The listing builds one solid part. Answer for the finished solid, in the listing's coordinates (mm). Face numbers are marked on the shaded views. A direction names the side the tool comes from. Round coordinates to 2 decimals unless told otherwise and drop trailing zeros. Order: outer loops, then holes, each group sorted by start corner. A loop starts at its lowest first (then second) coordinate and runs counter-clockwise, first axis right, second up. Notation, with made-up numbers: (-20.75, -12) -> (35.25, -12) arc R21 cw to (35.25, 17) -> close; hole circle Ø4 at (3, 56). An arc over 180 degrees is marked (long way). Answer in a Markdown table with one row per item. Add a question column.
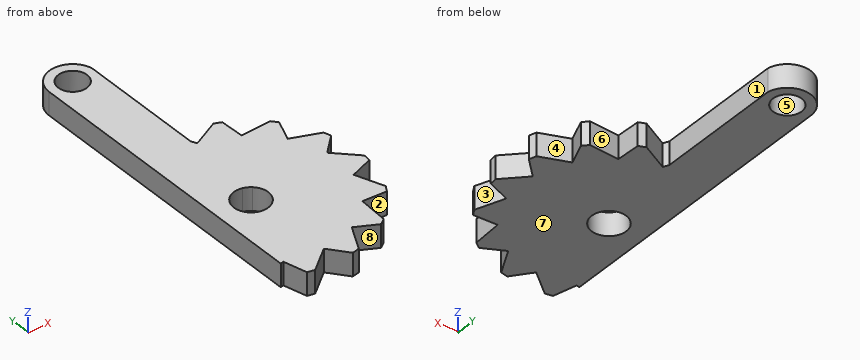
```python
from build123d import *

# Parameters (mm, degrees)
SKETCH1_R           = 1.25
BOSS_EXTRUDE2_DEPTH = 2


with BuildPart() as part:
    # Sketch1 → Boss-Extrude2 (new body)
    with BuildSketch(Plane.XY):
        with BuildLine():
            Line((8.285184221, -4.420298479), (7.377074087, -2.008607594))
            Line((7.377074087, -2.008607594), (9.301041093, -1.293812508))
            Line((9.301041093, -1.293812508), (9.366789776, -0.66825558))
            Line((9.366789776, -0.66825558), (7.556266833, 1.165572006))
            Line((7.556266833, 1.165572006), (9.023164798, 2.601117692))
            Line((9.023164798, 2.601117692), (8.828792284, 3.199334781))
            Line((8.828792284, 3.199334781), (6.428912397, 4.138213618))
            Line((6.428912397, 4.138213618), (7.185101337, 6.046291012))
            Line((7.185101337, 6.046291012), (6.764216399, 6.513731092))
            Line((6.764216399, 6.513731092), (4.189940603, 6.3953205))
            Line((4.189940603, 6.3953205), (4.10466858, 8.446005688))
            Line((4.10466858, 8.446005688), (3.530046047, 8.701844123))
            Line((3.530046047, 8.701844123), (1.226490014, 7.546618369))
            Line((1.226490014, 7.546618369), (1, 8.003257429))
            Line((1, 8.003257429), (1, 19))
            ThreePointArc((1, 19), (-1.19198009, 20.624419756), (-3.040958638, 18.618230684))
            Line((-3.040958638, 18.618230684), (-3.040958638, -7.197788875))
            Line((-3.040958638, -7.197788875), (-2.76871845, -7.126705038))
            Line((-2.76871845, -7.126705038), (-2.2589484, -9.114848784))
            Line((-2.2589484, -9.114848784), (-1.643690947, -9.245625793))
            Line((-1.643690947, -9.245625793), (0.36934192, -7.636708264))
            Line((0.36934192, -7.636708264), (1.643690947, -9.245625793))
            Line((1.643690947, -9.245625793), (2.2589484, -9.114848784))
            Line((2.2589484, -9.114848784), (3.443539717, -6.826255253))
            Line((3.443539717, -6.826255253), (5.262121196, -7.777750108))
            Line((5.262121196, -7.777750108), (5.770995046, -7.408031615))
            Line((5.770995046, -7.408031615), (5.922318213, -4.835480694))
            Line((5.922318213, -4.835480694), (7.970682886, -4.965030771))
            Line((7.970682886, -4.965030771), (8.285184221, -4.420298479))
        make_face()
        with BuildLine():
            ThreePointArc((0.384303163, 1.449934853), (0.711767769, 1.320373675), (1, 1.118033989))
            ThreePointArc((1, 1.118033989), (-0.706323533, -1.323294021), (0.372346585, 1.45305128))
            Line((0.372346585, 1.45305128), (0.384303163, 1.449934853))
        make_face(mode=Mode.SUBTRACT)
        with Locations((-1, 18.592345483)):
            Circle(SKETCH1_R, mode=Mode.SUBTRACT)
    extrude(amount=BOSS_EXTRUDE2_DEPTH)


solid = part.part
```
1. The part is cut by section A-A (x = -1). Give the vertices of the cut face in (y, z).
2. The part is cut by section D-D (y = 10.5). Give the vertices of the cut face in (x, z), then the cut area to 3 significant figures.
3. The part is cut by section B-B (y = 0). Give the vertices of the cut face in (x, z), then the cut area to 3 significant figures.
4. Each of these flat-tipped pins is pushed along its axis until it touches: pin 1 (1 mm diameter, centred on x = 0, y = 15, fed in from -Z); pin 2 (1 mm diameter, centred on x = 7.5, z = 1.5, fed in from +Y). Where does it stop, or does it pass through?
5. The part is cut by section C-C (z = 0.3). Give the number of separate pieces and of enclosed holes in the cut face, then the cut area to 3 significant figures.
6. Straight lines are drawn through the part: line 1 along Y through (x, z) = (-1, 1.5); line 2 along X through (y, z) = (18.5, 1.35); line 3 along Y through (x, z) = (0, 1.1). For each, find the intervals that lie inside material, in ascending order.
7. For the marked faces 4, 5, 6, 7 and 8, determine the directions among +Z, -Z, +X, -X, +Y, -Y from which every point of the face is accessible in a straight line to the end or side of a thin tool.
8. The mould has two halves that part along Y. Classify the marked faces 1, 2 and 3: released by +Y, released by -Y, zero draft, split by the parting line, or undercut.
Report:
| question | item | result |
|---|---|---|
| 1 | outline | (-8.73, 0) -> (-1.12, 0) -> (-1.12, 2) -> (-8.73, 2) -> close; (1.12, 0) -> (17.34, 0) -> (17.34, 2) -> (1.12, 2) -> close; (19.84, 0) -> (20.63, 0) -> (20.63, 2) -> (19.84, 2) -> close |
| 2 | outline | (-3.04, 0) -> (1, 0) -> (1, 2) -> (-3.04, 2) -> close |
| 2 | area | 8.08 mm^2 |
| 3 | outline | (-3.04, 0) -> (-1.5, 0) -> (-1.5, 2) -> (-3.04, 2) -> close; (1.5, 0) -> (8.71, 0) -> (8.71, 2) -> (1.5, 2) -> close |
| 3 | area | 17.5 mm^2 |
| 4 | pin 1 | stops at z = 0 |
| 4 | pin 2 | stops at y = 6.25 |
| 5 | separate pieces | 1 |
| 5 | enclosed holes | 2 |
| 5 | area | 203 mm^2 |
| 6 | line 1 | y = -8.73 to -1.12, 1.12 to 17.34, 19.84 to 20.63 |
| 6 | line 2 | x = -3.04 to -2.25, 0.25 to 1 |
| 6 | line 3 | y = -7.93 to -1.5, 1.5 to 17.84, 19.34 to 20.37 |
| 7 | face 4 | +Z, -Z, +X |
| 7 | face 5 | +Z, -Z |
| 7 | face 6 | +Z, -Z, +Y |
| 7 | face 7 | -Z, +X, -X, +Y, -Y |
| 7 | face 8 | +Z, -Z, -Y |
| 8 | face 1 | zero draft |
| 8 | face 2 | released by -Y |
| 8 | face 3 | undercut |
